```python
from build123d import *

# Parameters (mm, degrees)
F1_DEPTH = 12.7
F2_W     = 32.6402336359
F2_H     = 28.2041579485
F3_DEPTH = 76.2
F4_W     = 22.6674545556
F4_H     = 12.7
F5_DEPTH = 38.608
F6_R     = 8.7685690735
F7_DEPTH = 76.2
F8_R     = 7.62
F9_SIZE  = 10


with BuildPart() as f1:
    # F0 (on Top) → F1 (new body)
    with BuildSketch(Plane.XY):
        Polygon((94.5960357785, 36.9925387204), (-43.2745479047, 36.9925387204), (-43.2745479047, -59.7194693983), (58.4955252707, -59.7194693983), (69.8579475284, -59.7194693983), (94.5960357785, -59.7194693983), (94.5960357785, -27.4753328413), (94.5960357785, -27.073610574), align=None)
    extrude(amount=F1_DEPTH)

    # F2 (on face) → F3 (join)
    with BuildSketch(Plane.XY.offset(12.7)):
        with Locations((78.2759189606, -45.617390424)):
            Rectangle(F2_W, F2_H)
    extrude(amount=-F3_DEPTH)

    # F4 (on face) → F5 (cut)
    with BuildSketch(Plane.YZ.offset(94.5960357785)):
        with Locations((25.6588114426, 6.35)):
            Rectangle(F4_W, F4_H)
    extrude(amount=-F5_DEPTH, mode=Mode.SUBTRACT)

    # F6 (on face) → F7 (cut)
    with BuildSketch(Plane(origin=(0, 0, -63.5), x_dir=(1, 0, 0), z_dir=(0, 0, -1))):
        with Locations((78.1861692667, 44.3040877581)):
            Circle(F6_R)
    extrude(amount=-F7_DEPTH, mode=Mode.SUBTRACT)

    # F8
    f8_edges = [f1.edges().sort_by_distance(p)[0] for p in [
        (-43.274548, 36.992539, 6.35),
    ]]
    fillet(f8_edges, radius=F8_R)

    # F9
    f9_edges = [f1.edges().sort_by_distance(p)[0] for p in [
        (-43.274548, -59.719469, 6.35),
    ]]
    chamfer(f9_edges, length=F9_SIZE)


solid = f1.part
```
Design review of the part built by this model. Coordinates are the model's own, in mm. A direction names the side the tool comes from. Round coordinates to 2 decimals unless told otherwise and drop trailing zeros. Write each loop counter-clockwise with the first axis right and the second up, starting at its lowest first coordinate (ties: lowest second). Pieces come first, ordered by that corner, then holes.
Item 1: We need section C-C on z = 4.5. Write out the cut boundary in (x, y).
Item 2: We need section B-B on x = 72. Write out the cut boundary in (y, z), and give its area (3 significant figures).
Item 3: The part is to be moulded in two halves that separate along Y. For faces 6 (the flat face through (11, 36.993, 6)), 7 (the cylindrical face through (86.29, -40.95, -25.93)), 8 (the flat face through (-43.275, -10, 6)), say which applies: +Y half, -Y half, draft (parallel to the pull), parting line (faces both ways), or undercut.
Item 4: We need section D-D on y = 19.5. Write out the cut boundary in (x, z), and give its area (3 significant figures).
Item 5: Clearance check with flat-ended pins moving along their axes: pin 1 Ø14 at (y, z) = (20, 7) entering from +X; pin 2 Ø14 at (x, z) = (79, 6.5) entering from +Y; pin 3 Ø2 at (x, y) = (3.5, -11) entering from -Z; pin 4 Ø22.5 at (y, z) = (-43, -45) entering from -X. State where each tip first meets the part, or that it passes through.
Item 6: For probe 1 along Z at (x, y) = (-20, -33); probe 2 along Y at (x, z) = (87, 8); probe 3 along Y at (x, z) = (75.5, -13), list the stretches that pass through material, from the lowest coordinate up.
Item 7: For faces 1 (the flat face through (61.956, -46, -31)), 2 (the flat face through (25, -11, 12.7)), 3 (the flat face through (78, -31.515, -31)), 4 (the flat face through (76, 14.325, 6)), 5 (the flat face through (94.596, -40, -17)), list the 3-axis set-ups (+Z, -Z, +X, -X, +Y, -Y) from which the entire face can be reached by the end or side of a thin tool; tool diameter is ignored.
Item 8: We need section A-A on y = -39. Write out the cut boundary in (x, z).
Returned:
1. outline: (-43.27, -49.72) - (-33.27, -59.72) - (94.6, -59.72) - (94.6, 14.33) - (55.99, 14.33) - (55.99, 36.99) - (-35.65, 36.99) arc R7.62 ccw to (-43.27, 29.37) - close; hole circle Ø17.54 at (78.19, -44.3)
2. outline: (-59.72, -63.5) - (-50.52, -63.5) - (-50.52, 12.7) - (-59.72, 12.7) - close; (-38.09, -63.5) - (-31.52, -63.5) - (-31.52, 0) - (14.33, 0) - (14.33, 12.7) - (-38.09, 12.7) - close
2. area: 1,780 mm2
3. face 6: +Y half
3. face 7: undercut
3. face 8: draft
4. outline: (-43.27, 0) - (55.99, 0) - (55.99, 12.7) - (-43.27, 12.7) - close
4. area: 1,260 mm2
5. pin 1: stops at x = 94.6
5. pin 2: stops at y = 14.33
5. pin 3: stops at z = 0
5. pin 4: stops at x = 61.96
6. probe 1: z = 0 to 12.7
6. probe 2: y = -59.72 to 14.33
6. probe 3: y = -59.72 to -52.65, -35.96 to -31.52
7. face 1: -Z, -X, +Y, -Y
7. face 2: +Z, +X, -X, +Y, -Y
7. face 3: -Z, +X, -X, +Y
7. face 4: +Z, -Z, +X, +Y
7. face 5: +Z, -Z, +X, +Y, -Y
8. outline: (-43.27, 0) - (61.96, 0) - (61.96, -63.5) - (71.2, -63.5) - (71.2, 12.7) - (-43.27, 12.7) - close; (85.17, -63.5) - (94.6, -63.5) - (94.6, 12.7) - (85.17, 12.7) - close
